Answer from the drawing. Dimensions are ordinates in mm from the lowest x, y and z of the part. Give positions to 0.01 mm unless a question says otherwise; leave off trailing zeros. Write each loop counter-clockwise with the first axis right and the second up, starting at its lowest first coordinate (ties: lowest second). Pieces come first, ordered by that corner, then holes.
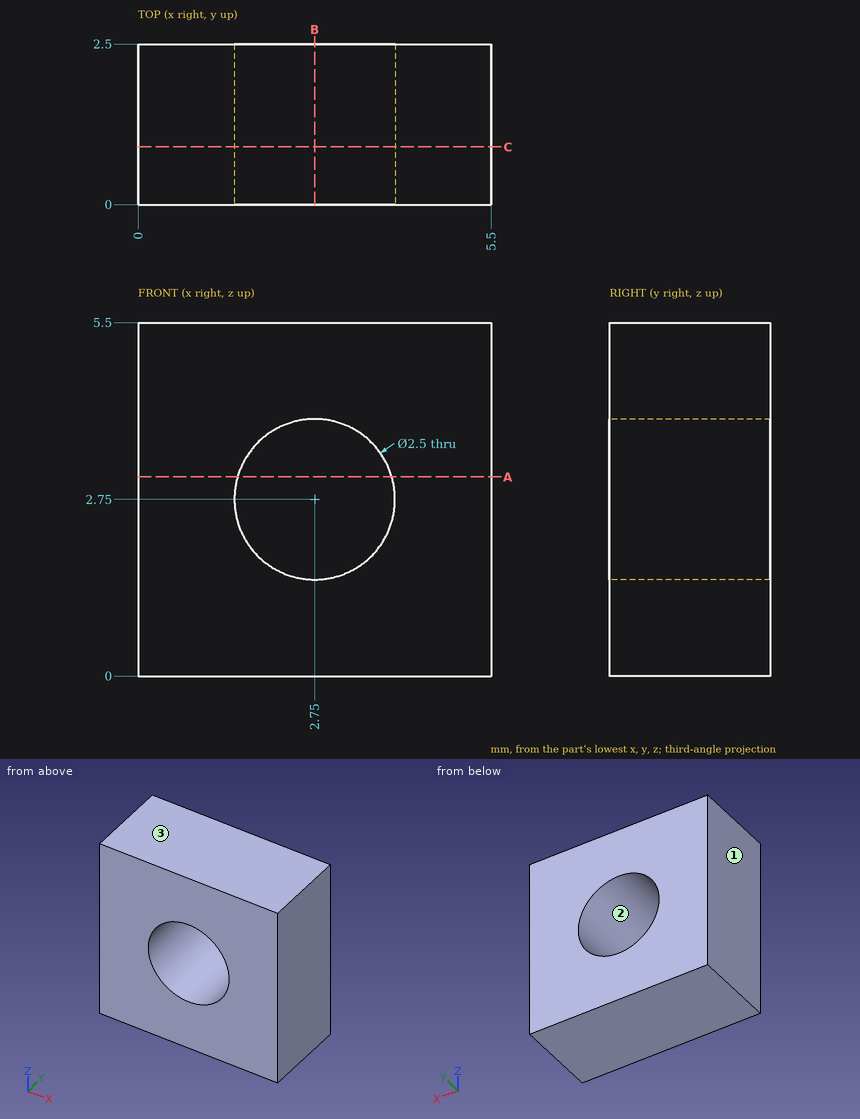
Item 1: Consider probe 1 along Z at (x, y) = (2.75, 1.75); probe 2 along X at (y, z) = (0.55, 2.05). Determine where each line is inside the solid, lowest interval first.
Conclusion:
probe 1: z = 0 to 1.5, 4 to 5.5
probe 2: x = 0 to 1.71, 3.79 to 5.5
Item 2: Determine the mould class of the marked faces 1, 2 and 3 for opening direction X: pulls with the +X half, pulls with the -X half, needs draft (parallel to the pull), parting line crosses it, or undercut.
Conclusion:
face 1: pulls with the -X half
face 2: undercut
face 3: needs draft
Item 3: A cutting plane is placed at B-B, the plane x = 2.75. Give the vertices of the cut face in (y, z).
Conclusion:
outline: (0, 0) - (2.5, 0) - (2.5, 1.5) - (0, 1.5) - close; (0, 4) - (2.5, 4) - (2.5, 5.5) - (0, 5.5) - close
Item 4: Each of these flat-tipped pins is pushed along its axis until it touches: P1, Ø1, axis at x = 2, z = 5, coming from the -Y side; P2, Ø2, axis at x = 2.75, z = 2.75, coming from the +Y side. Where does it stop, or does it pass through?
Conclusion:
P1: stops at y = 0
P2: passes through
Item 5: A cutting plane is placed at A-A, the plane z = 3.1. Give the vertices of the cut face in (x, y).
Conclusion:
outline: (0, 0) - (1.55, 0) - (1.55, 2.5) - (0, 2.5) - close; (3.95, 0) - (5.5, 0) - (5.5, 2.5) - (3.95, 2.5) - close
Item 6: A cutting plane is placed at C-C, the plane y = 0.9. Give the vertices of the cut face in (x, z).
Conclusion:
outline: (0, 0) - (5.5, 0) - (5.5, 5.5) - (0, 5.5) - close; hole circle Ø2.5 at (2.75, 2.75)
